from build123d import *

# Parameters (mm, degrees)
F0_W      = 126.798056066
F0_H      = 64.8966394365
F1_DEPTH  = 25.4
F3_DEPTH  = 25.4
F4_W      = 47.5243106484
F4_H      = 30.5513413623
F5_DEPTH  = 10.16
F6_W      = 47.5243106484
F6_H      = 15.3855457902
F7_DEPTH  = 20.32
F8_W      = 36.6652142256
F8_H      = 13.0012265766
F9_DEPTH  = 25.4
F10_W     = 10.1351421326
F10_H     = 15.3855457902
F11_DEPTH = 15.24
F12_W     = 10.8590964228
F12_H     = 15.1657955721
F13_DEPTH = 7.62
F15_DEPTH = 43.18
F17_DEPTH = 50.8


with BuildPart() as f1:
    # F0 (on Top) → F1 (new body)
    with BuildSketch(Plane.XY):
        with Locations((0.8286423981, -17.062773928)):
            Rectangle(F0_W, F0_H)
    extrude(amount=F1_DEPTH)

    # F2 (on face) → F3 (cut)
    with BuildSketch(Plane.XY.offset(25.4)):
        Polygon((-23.0333544314, -49.5110936463), (-62.5703856349, -2.7855145745), (-62.5703856349, -49.5110936463), align=None)
        Polygon((64.2276704311, -2.9851964209), (24.2912732065, -49.5110936463), (64.2276704311, -49.5110936463), align=None)
    extrude(amount=-F3_DEPTH, mode=Mode.SUBTRACT)

    # F4 (on face) → F5 (join)
    with BuildSketch(Plane.XY.offset(25.4)):
        with Locations((-2.8654746711, 0.109875109)):
            Rectangle(F4_W, F4_H)
    extrude(amount=F5_DEPTH)

    # F6 (on face) → F7 (join)
    with BuildSketch(Plane.XY.offset(35.56)):
        with Locations((-2.8654746711, 7.6927728951)):
            Rectangle(F6_W, F6_H)
    extrude(amount=F7_DEPTH)

    # F8 (on face) → F9 (cut)
    with BuildSketch(Plane.XZ):
        with Locations((2.5640735403, 42.0606132883)):
            Rectangle(F8_W, F8_H)
    extrude(amount=-F9_DEPTH, mode=Mode.SUBTRACT)

    # F10 (on face) → F11 (cut)
    with BuildSketch(Plane.XY.offset(55.88)):
        with Locations((15.8291095868, 7.6927728951)):
            Rectangle(F10_W, F10_H)
    extrude(amount=-F11_DEPTH, mode=Mode.SUBTRACT)

    # F12 (on face) → F13 (join)
    with BuildSketch(Plane.XY.offset(35.56)):
        with Locations((-21.198081784, -7.5828977861)):
            Rectangle(F12_W, F12_H)
    extrude(amount=F13_DEPTH)

    # F14 (on face) → F15 (cut)
    with BuildSketch(Plane.XY.offset(25.4)):
        with BuildLine():
            Line((-55.6119495793, 1.3946691004), (-44.2270040512, 0))
            Line((-44.2270040512, 0), (-42.8323349509, 11.3849455281))
            ThreePointArc((-42.8323349509, 11.3849455281), (-51.2911962592, 9.0365521647), (-55.6119495793, 1.3946691004))
        make_face()
        with BuildLine():
            Line((-44.2270040512, -11.4700517251), (-44.2270040512, 0))
            Line((-44.2270040512, 0), (-55.6119495793, 1.3946691004))
            ThreePointArc((-55.6119495793, 1.3946691004), (-52.8165038416, -7.6014853764), (-44.2270040512, -11.4700517251))
        make_face()
        with BuildLine():
            Line((-32.8420585231, -1.3946691004), (-44.2270040512, 0))
            Line((-44.2270040512, 0), (-44.2270040512, -11.4700517251))
            ThreePointArc((-44.2270040512, -11.4700517251), (-36.6255186748, -8.5894997904), (-32.8420585231, -1.3946691004))
        make_face()
        with BuildLine():
            Line((-42.8323349509, 11.3849455281), (-44.2270040512, 0))
            Line((-44.2270040512, 0), (-32.8420585231, -1.3946691004))
            ThreePointArc((-32.8420585231, -1.3946691004), (-32.7782486457, -0.698631692), (-32.7569523261, 0))
            ThreePointArc((-32.7569523261, 0), (-35.6375042608, 7.6014853764), (-42.8323349509, 11.3849455281))
        make_face()
    extrude(amount=-F15_DEPTH, mode=Mode.SUBTRACT)

    # F16 (on face) → F17 (cut)
    with BuildSketch(Plane.XY.offset(25.4)):
        with BuildLine():
            Line((39.2047164649, -0.6157344434), (45.6754229963, 0))
            Line((45.6754229963, 0), (45.0596885529, 6.4707065314))
            ThreePointArc((45.0596885529, 6.4707065314), (40.6645525286, 4.1400904671), (39.2047164649, -0.6157344434))
        make_face()
        with BuildLine():
            Line((45.0596885529, 6.4707065314), (45.6754229963, 0))
            Line((45.6754229963, 0), (51.6652548153, 2.5241011666))
            ThreePointArc((51.6652548153, 2.5241011666), (49.0092127508, 5.5798761449), (45.0596885529, 6.4707065314))
        make_face()
        with BuildLine():
            Line((51.6652548153, 2.5241011666), (45.6754229963, 0))
            Line((45.6754229963, 0), (46.2911574396, -6.4707065314))
            ThreePointArc((46.2911574396, -6.4707065314), (50.4843421358, -4.3730388324), (52.1753592975, 0))
            ThreePointArc((52.1753592975, 0), (52.0465570083, 1.2875648801), (51.6652548153, 2.5241011666))
        make_face()
        with BuildLine():
            Line((46.2911574396, -6.4707065314), (45.6754229963, 0))
            Line((45.6754229963, 0), (39.2047164649, -0.6157344434))
            ThreePointArc((39.2047164649, -0.6157344434), (41.5353325292, -5.0108704677), (46.2911574396, -6.4707065314))
        make_face()
    extrude(amount=-F17_DEPTH, mode=Mode.SUBTRACT)


solid = f1.part
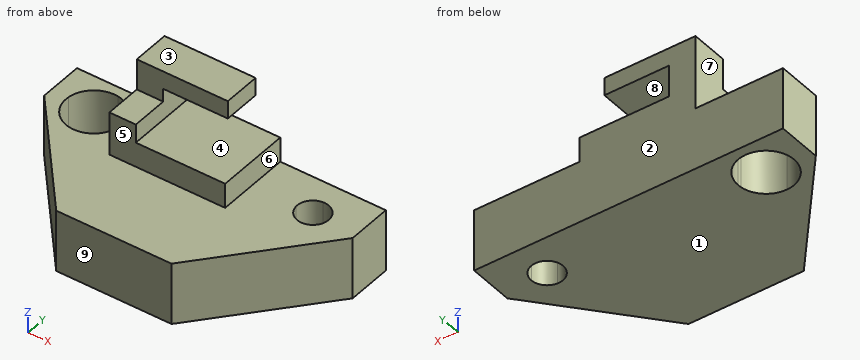
Build history of the part. All positions in model axes, mm. Face numbers are marked on the shaded views. A direction names the side the tool comes from. Give positions to 0.01 mm unless a question says otherwise; leave off trailing zeros. Loops run counter-clockwise (first coordinate to the right, second up) from the corner with the lowest first, then second, coordinate; pieces in that order, holes last. Notation, with made-up numbers: (56.25, 51.5) - (108.25, 51.5) arc R26 ccw to (108.25, 82.5) - close; hole circle Ø4 at (-20.5, 46.25). An arc over 180 degrees is marked (long way). Write item = value, one per line. Start each with the question number.
1) Band-saw the part on A-A on x = -18. Give the cut face in (y, z).
2) Tool access for the marked faces 5, 6, 7, 8 and 9: list every direction of +Z, -Z, +X, -X, +Y, -Y with a clear straight run to the whole face (end or side of a thin tool).
3) Probe probe 1 along Z at (x, y) = (12.5, -39); probe 2 along X at (y, z) = (-3, 15); probe 3 along Z at (x, y) = (17, -9.5). List the from-to ranges inside material, lowest first. Write a range as from..to.
4) Band-saw the part on B-B on z = 16. Give the cut face in (x, y), plus the area to 3 significant figures.
5) Band-saw the part on D-D on y = -19. Give the cut face in (x, z).
6) Band-saw the part on C-C on z = 27.5. Give the cut face in (x, y), plus the area to 3 significant figures.
7) Pull direction Z, two halves, no side cores. Call the marked faces 1, 2, 3 and 4: +Z half, -Z half, draft (parallel to the pull), parting line (faces both ways), or undercut.
8) Drop flat-ended pins along their axis: pin 1 Ø5 at (y, z) = (-1, 30.5) entering from +X; pin 2 Ø4 at (x, z) = (17, 36.5) entering from +Y; pin 3 Ø1 at (x, y) = (5, -29) entering from +Z; pin 4 Ø2 at (y, z) = (-7.5, 29.5) entering from -X. Give the stop position or say it passes through.
Final values:
q1.outline = (-49.51, 0) - (15.39, 0) - (15.39, 55.88) - (0, 55.88) - (0, 43.18) - (-15.17, 43.18) - (-15.17, 25.4) - (-49.51, 25.4) - close
q2.face_5 = +Z, +X, -X, -Y
q2.face_6 = +Z, +X, +Y, -Y
q2.face_7 = +Z, -X, +Y, -Y
q2.face_8 = +X, +Y, -Y
q2.face_9 = +Z, -Z, +X, -X, -Y
q3.probe_1 = 0..25.4
q3.probe_2 = -62.39..-55.3, -33.16..39.91, 51.44..64.21
q3.probe_3 = 0..35.56
q4.outline = (-62.57, -2.79) - (-23.03, -49.51) - (24.29, -49.51) - (64.23, -2.99) - (64.23, 15.39) - (-62.57, 15.39) - close; hole circle Ø22.94 at (-44.23, 0); hole circle Ø13 at (45.68, 0)
q4.area = 5,830 mm²
q5.outline = (-48.85, 0) - (50.48, 0) - (50.48, 25.4) - (-48.85, 25.4) - close
q6.outline = (-26.63, -15.17) - (20.9, -15.17) - (20.9, 15.39) - (-26.63, 15.39) - close
q6.area = 1,450 mm²
q7.face_1 = -Z half
q7.face_2 = draft
q7.face_3 = +Z half
q7.face_4 = undercut
q8.pin_1 = 20.9
q8.pin_2 = 15.39
q8.pin_3 = 25.4
q8.pin_4 = -26.63
